from build123d import *

# Parameters (mm, degrees)
SKETCH2_W           = 24.75
SKETCH2_H           = 4
BOSS_EXTRUDE1_DEPTH = 10
SKETCH3_R           = 0.5
CUT_EXTRUDE1_DEPTH  = 5


with BuildPart() as part:
    # Sketch2 → Boss-Extrude1 (new body)
    with BuildSketch(Plane.XY):
        with Locations((12.375, 2)):
            Rectangle(SKETCH2_W, SKETCH2_H)
    extrude(amount=BOSS_EXTRUDE1_DEPTH)

    # Sketch3 → Cut-Extrude1 (cut)
    with BuildSketch(Plane.XY.offset(10)):
        with Locations((1.125, 2)):
            Circle(SKETCH3_R)
        with Locations((2.375, 2)):
            Circle(SKETCH3_R)
        with Locations((3.625, 2)):
            Circle(SKETCH3_R)
        with Locations((4.875, 2)):
            Circle(SKETCH3_R)
        with Locations((6.125, 2)):
            Circle(SKETCH3_R)
        with Locations((7.375, 2)):
            Circle(SKETCH3_R)
        with Locations((8.625, 2)):
            Circle(SKETCH3_R)
        with Locations((9.875, 2)):
            Circle(SKETCH3_R)
        with Locations((11.125, 2)):
            Circle(SKETCH3_R)
        with Locations((12.375, 2)):
            Circle(SKETCH3_R)
        with Locations((13.625, 2)):
            Circle(SKETCH3_R)
        with Locations((14.875, 2)):
            Circle(SKETCH3_R)
        with Locations((16.125, 2)):
            Circle(SKETCH3_R)
        with Locations((17.375, 2)):
            Circle(SKETCH3_R)
        with Locations((18.625, 2)):
            Circle(SKETCH3_R)
        with Locations((19.875, 2)):
            Circle(SKETCH3_R)
        with Locations((21.125, 2)):
            Circle(SKETCH3_R)
        with Locations((22.375, 2)):
            Circle(SKETCH3_R)
        with Locations((23.625, 2)):
            Circle(SKETCH3_R)
    extrude(amount=-CUT_EXTRUDE1_DEPTH, mode=Mode.SUBTRACT)


solid = part.part
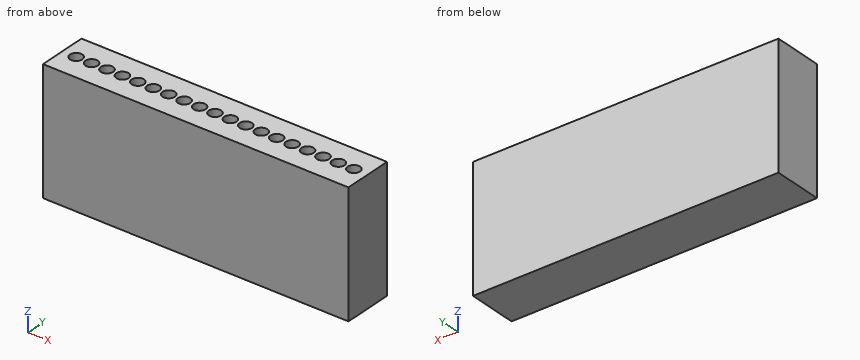
Design review of the part built by this model. Coordinates are the model's own, in mm. Give positions to 0.01 mm unless a question says otherwise; leave off trailing zeros. Order: outer loops, then holes, each group sorted by start corner. A loop starts at its lowest first (then second) coordinate and runs counter-clockwise, first axis right, second up. Notation, with made-up numbers: (86, 21.25) - (131, 21.25) arc R22 ccw to (131, 50.25) - close; hole circle Ø10 at (-27.75, 76). An arc over 180 degrees is marked (long way). Write item = value, one per line. Start each with the question number.
Q1. Clearance check with a flat-ended pin moving along its axis: pin 1 Ø0.5 at (x, y) = (10, 2) entering from +Z. State where the tip first meets the part, or that it passes through.
Q2. To check wall thickness, follow L1, parallel to Z at x = 5, y = 1.65; L2, parallel to Y at x = 19, z = 8.25. State the ranges of each line that lie inside material, in increasing order. Write a range as from..to.
Q3. We need section B-B on x = 11. State the section outline as (y, z) points, plus the area to 3 significant figures.
Q4. We need section A-A on z = 8.25. State how many separate pieces and enclosed holes the cut face has, plus the area to 3 significant figures.
Working result:
q1.pin_1 = 5
q2.L1 = 0..5
q2.L2 = 0..1.67, 2.33..4
q3.outline = (0, 0) - (4, 0) - (4, 10) - (2.48, 10) - (2.48, 5) - (1.52, 5) - (1.52, 10) - (0, 10) - close
q3.area = 35.2 mm²
q4.separate_pieces = 1
q4.enclosed_holes = 19
q4.area = 84.1 mm²
